```python
from build123d import *

# Parameters (mm, degrees)
SKETCH_1_W      = 8
SKETCH_1_H      = 3
EXTRUDE_1_DEPTH = 3


with BuildPart() as part:
    # 草图1 → 凸台-拉伸1 (new body)
    with BuildSketch(Plane.XY):
        Polygon((38, 0), (-38, 0), (-38, -25), (-41, -25), (-41, -33), (-38, -33), (-38, -41), (-31, -41), (-31, -51), (-30, -51), (-30, -54), (-22, -54), (-22, -51), (-14, -51), (-14, -33), (14, -33), (14, -51), (22, -51), (22, -54), (30, -54), (30, -51), (31, -51), (31, -41), (38, -41), (38, -33), (41, -33), (41, -25), (38, -25), align=None)
        with Locations((26, -31.5)):
            Rectangle(SKETCH_1_W, SKETCH_1_H, mode=Mode.SUBTRACT)
        with Locations((-26, -31.5)):
            Rectangle(SKETCH_1_W, SKETCH_1_H, mode=Mode.SUBTRACT)
    extrude(amount=EXTRUDE_1_DEPTH)


solid = part.part
```
Here's how the part is built. I have some questions about the finished solid (model axes, mm). A direction names the side the tool comes from. Coordinates: 2 decimals unless noted, no trailing zeros. Order: outer loops, then holes, each group sorted by start corner. A loop starts at its lowest first (then second) coordinate and runs counter-clockwise, first axis right, second up.
Item 1: If we section it at C-C, the plane z = 2.4: Give the number of separate pieces and of enclosed holes in the cut face, then the cut area to 3 significant figures.
Response values:
separate pieces: 1
enclosed holes: 2
area: 3,280 mm2
Item 2: Which directions (+Z, -Z, +X, -X, +Y, -Y) give clear straight access to the entire face, cutting with the end or side of a thin tool? Please do faces 1 (the face through (-26, -33, 1)), 2 (the face through (-30, -52, 1)), 3 (the face through (-22, -53, 1)), 4 (the face through (41, -29, 1)), 5 (the face through (34, -41, 1)).
Response values:
face 1: +Z, -Z
face 2: +Z, -Z, -X, -Y
face 3: +Z, -Z, -Y
face 4: +Z, -Z, +X, +Y, -Y
face 5: +Z, -Z, +X, -Y
Item 3: If we section it at D-D, the plane y = -3.5: List the corners of the cut face in (x, z) for me.
Response values:
outline: (-38, 0) - (38, 0) - (38, 3) - (-38, 3) - close
Item 4: I'm going to push flat-ended pins straight in: pin 1 Ø1.5 at (x, z) = (17.5, 2) entering from -Y; pin 2 Ø1.5 at (y, z) = (-37.5, 1) entering from -X; pin 3 Ø0.9 at (x, z) = (-39.5, 1) entering from +Y. Where does each tip first touch, or does it pass through?
Response values:
pin 1: stops at y = -51
pin 2: stops at x = -38
pin 3: stops at y = -25
Item 5: If we section it at A-A, the plane y = -42: List the corners of the cut face in (x, z) for me, then the cut area to 3 significant figures.
Response values:
outline: (-31, 0) - (-14, 0) - (-14, 3) - (-31, 3) - close; (14, 0) - (31, 0) - (31, 3) - (14, 3) - close
area: 102 mm2
Item 6: I need wall thicknesses on probe 1 along X at (y, z) = (-32.5, 1.4); probe 2 along Y at (x, z) = (16, 2.1); probe 3 along X at (y, z) = (-24.5, 2.55). Which ranges of each line are inside material? Lowest first, please.
Response values:
probe 1: x = -41 to -30, -22 to 22, 30 to 41
probe 2: y = -51 to 0
probe 3: x = -38 to 38
Item 7: If we section it at B-B, the plane x = -27.5: List the corners of the cut face in (y, z) for me, then the cut area to 3 significant figures.
Response values:
outline: (-54, 0) - (-33, 0) - (-33, 3) - (-54, 3) - close; (-30, 0) - (0, 0) - (0, 3) - (-30, 3) - close
area: 153 mm2
Item 8: Thinking about a two-plate mould opening in Y: for faces 6 (the face through (40, -25, 1)), 7 (the face through (38, -13, 1)), 8 (the face through (26, -33, 1)), which applies, pulls with the +Y half, pulls with the -Y half, needs draft (parallel to the pull), parting line crosses it, or undercut?
Response values:
face 6: pulls with the +Y half
face 7: needs draft
face 8: undercut
